Geometry check sheet. Reference: the model listing, model coordinates, mm. A direction names the side the tool comes from. Give positions to 0.01 mm unless a question says otherwise; leave off trailing zeros. Order: outer loops, then holes, each group sorted by start corner. A loop starts at its lowest first (then second) coordinate and runs counter-clockwise, first axis right, second up. Notation, with made-up numbers: M 82.5,57.25 L 137.5,57.25 A18 ccw 137.5,84.25 Z; hole C -32.75,18 d10. An arc over 180 degrees is marked long. Put each result on its own line as item: value. Start each with the question number.
Q1. Go/stop test with flat-tipped pins: pin 1 (0.5 mm diameter, centred on x = 1, y = -21, fed in from -Z); pin 2 (0.8 mm diameter, centred on x = 0.5, z = -13.5, fed in from -Y). Record where each tip stops, or that it passes through.
Q2. Material ranges on L1, parallel to Z at x = 0.35, y = 16.5; L2, parallel to Y at x = 1.45, z = -12.75; L3, parallel to Z at x = 0.7, y = -8, recorded low to high.
Q3. Section check B-B on z = -2.75. Record the cut outline in (x, y), then the cut area to 3 significant figures.
Q4. Access from +Z, -Z, +X, -X, +Y, -Y to the whole of each face (thin tool, end or side, straight path). Record for faces 1 (the flat face through (1, -4.762, -13)), 2 (the flat face through (1, 4.762, -13)), 3 (the flat face through (1, 0, -14.288)).
Q5. Section check A-A on y = 26.5. Record the cut outline in (x, z), then the cut area to 3 significant figures.
```python
from build123d import *

# Parameters (mm, degrees)
SKETCH2_W           = 25.4
SKETCH2_H           = 63.5
BOSS_EXTRUDE1_DEPTH = 1.5875
SKETCH3_W           = 1.5875
SKETCH3_H           = 9.525
BOSS_EXTRUDE2_DEPTH = 1.5875
SKETCH3_4_W         = 1.5875
SKETCH3_4_H         = 9.525
CUT_EXTRUDE1_DEPTH  = 3.175
CUT_EXTRUDE2_DEPTH  = 35.85276621
CAVITY1_OUTLINE_W   = 13.081
CAVITY1_OUTLINE_H   = 49.289563405


# Read off the part's stored shape, not the designer's step: Cavity1
with BuildPart() as part:
    # Sketch2 → Boss-Extrude1 (new body)
    with BuildSketch(Plane(origin=(0, 0, 0), x_dir=(0, 0, -1), z_dir=(1, 0, 0))):
        Rectangle(SKETCH2_W, SKETCH2_H)
    extrude(amount=BOSS_EXTRUDE1_DEPTH)

    # Sketch3 → Boss-Extrude2 (add)
    with BuildSketch(Plane(origin=(1.5875, 0, 0), x_dir=(0, 0, -1), z_dir=(1, 0, 0))):
        with Locations((13.49375, 0)):
            Rectangle(SKETCH3_W, SKETCH3_H)
    extrude(amount=-BOSS_EXTRUDE2_DEPTH)

    # Sketch3<4> → Cut-Extrude1 (cut)
    with BuildSketch(Plane(origin=(1.5875, 0, 0), x_dir=(0, 0, -1), z_dir=(1, 0, 0))):
        with Locations((-11.90625, 0)):
            Rectangle(SKETCH3_4_W, SKETCH3_4_H)
    extrude(amount=-CUT_EXTRUDE1_DEPTH, mode=Mode.SUBTRACT)

    # Sketch4 → Cut-Extrude2 (cut, through all)
    with BuildSketch(Plane(origin=(1.5875, 0, 0), x_dir=(0, 0, -1), z_dir=(1, 0, 0))):
        Polygon((-6.14934, 31.75), (-6.14934, -31.75), (-12.7, -31.75), (-12.7, -4.7625), (-11.1125, -4.7625), (-11.1125, 4.7625), (-12.7, 4.7625), (-12.7, 31.75), align=None)
    extrude(amount=-CUT_EXTRUDE2_DEPTH, mode=Mode.SUBTRACT)

    # Cavity1 outline → Cavity1 (revolve, cut)
    with BuildSketch(Plane(origin=(-10.964254269, -1.274913287, 6.150528853), x_dir=(0.9933073803012532, 0.11550085817456804, 0), z_dir=(0, 0, -1))):
        with Locations((6.5405, 7.076085234)):
            Rectangle(CAVITY1_OUTLINE_W, CAVITY1_OUTLINE_H)
    revolve(axis=Axis((-10.964254269, -1.274913287, 6.150528853), (0.11550085817456807, -0.9933073803012534, 0)), mode=Mode.SUBTRACT)


solid = part.part
```
Results found:
1. pin 1: stops at z = -12.7
1. pin 2: stops at y = -4.76
2. L1: z = -12.7 to 6.15
2. L2: y = -4.76 to 4.76
2. L3: z = -12.7 to -1.22
3. outline: M 0,-12.57 L 1.59,-26.22 L 1.59,31.75 L 0,31.75 Z
3. area: 81.2 mm^2
4. face 1: -Z, +X, -X, -Y
4. face 2: -Z, +X, -X, +Y
4. face 3: -Z, +X, -X, +Y, -Y
5. outline: M 0,-12.7 L 1.59,-12.7 L 1.59,6.15 L 0,6.15 Z
5. area: 29.9 mm^2
